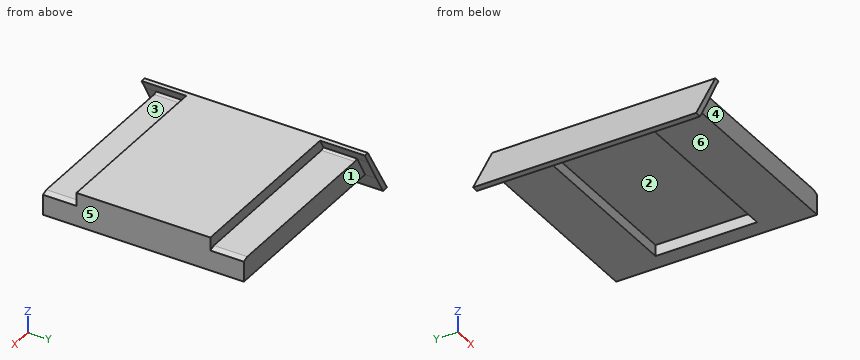
from build123d import *

# Parameters (mm, degrees)
F1_DEPTH  = 20
F3_DEPTH  = 4
F5_DEPTH  = 1
F7_DEPTH  = 20.001
F10_W     = 15
F10_H     = 9.1
F11_DEPTH = 1


# Not quite as in the source:
# - a pattern or mirror of a feature is missing from the dataset's text; its kind, count and spacing are read off the source's solid


with BuildPart() as f1:
    # F0 (on Front) → F1 (new body)
    with BuildSketch(Plane.XZ):
        Polygon((-16.45, 3), (-19.25, -1.7), (-18.09, -1.7), (-17.0772340426, 0), (0, 0), (0, 3), align=None)
    extrude(amount=F1_DEPTH)

    # F2 (on face) → F3 (cut)
    with BuildSketch(Plane.XZ.offset(20)):
        Polygon((-16.2, 2), (-0.5, 2), (0, 1.8180148829), (0, 3), (-16, 3), (-16.5, 2.1091910703), align=None)
    f3 = extrude(amount=-F3_DEPTH, mode=Mode.SUBTRACT)

    # F3_copies: F3 across plane
    add(f3.mirror(Plane.ZX.offset(-10)), mode=Mode.SUBTRACT)

    # F4 (on face) → F5 (cut)
    with BuildSketch(Plane.XZ.offset(20)):
        Polygon((0, 0), (0, 1.8180148829), (-0.5, 2), (-16.2, 2), (-16.5, 2.1091910703), (-17.683862779, 0), align=None)
    f5 = extrude(amount=-F5_DEPTH, mode=Mode.SUBTRACT)

    # F5_copies: F5 across plane
    add(f5.mirror(Plane.ZX.offset(-10)), mode=Mode.SUBTRACT)

    # F6 (on face) → F7 (cut, through all)
    with BuildSketch(Plane.XZ.offset(20)):
        Polygon((-18.67, -1.7), (-18.09, -1.7), (-17.0772340426, 0), (-17.683862779, 0), align=None)
    extrude(amount=-F7_DEPTH, mode=Mode.SUBTRACT)

    # F10 (on face) → F11 (cut)
    with BuildSketch(Plane(origin=(0, 0, 0), x_dir=(1, 0, 0), z_dir=(0, 0, -1))):
        with Locations((-9, 10)):
            Rectangle(F10_W, F10_H)
    extrude(amount=-F11_DEPTH, mode=Mode.SUBTRACT)


solid = f1.part
Could you check a few things on this model? Use its own coordinates, in mm. Face numbers are marked on the shaded views. A direction names the side the tool comes from. Coordinates: 2 decimals unless noted, no trailing zeros. Write each loop counter-clockwise with the first axis right and the second up, starting at its lowest first coordinate (ties: lowest second). Pieces come first, ordered by that corner, then holes. Notation, with made-up numbers: (-20, 65) - (-9, 65) arc R17 cw to (-9, 92) - close; hole circle Ø8 at (18.5, -39.5). An arc over 180 degrees is marked (long way). Write item = value, one per line.
1) For the marked faces 5 and 6, which set-ups out of +Z, -Z, +X, -X, +Y, -Y let a thin tool reach every point of the face, with its end or its side?
Result set:
face_5 = +Z, -Z, +X, +Y, -Y
face_6 = -Z, +X, +Y, -Y
2) Suppose I cut it at B-B on x = -8.75. Please give me the cut outline in (y, z).
Result set:
outline = (-19, 0) - (-14.55, 0) - (-14.55, 1) - (-5.45, 1) - (-5.45, 0) - (-1, 0) - (-1, 2) - (-4, 2) - (-4, 3) - (-16, 3) - (-16, 2) - (-19, 2) - close
3) Will these pins go through, and if not, where does the flat tip stop? pin 1 Ø2.5 at (x, y) = (-9, -8) entering from -Z; pin 2 Ø2.5 at (x, z) = (-10, 0.5) entering from +Y; pin 3 Ø0.6 at (x, z) = (-6.5, 2.5) entering from -Y.
Result set:
pin_1 = 1
pin_2 = -1
pin_3 = -16
4) We'd pull the mould along Y, two halves only. Please class the marked faces 1, 2, 3 and 4: +Y half, -Y half, draft (parallel to the pull), parting line (faces both ways), or undercut.
Result set:
face_1 = +Y half
face_2 = undercut
face_3 = draft
face_4 = -Y half
5) Suppose I cut it at A-A on y = -7.25. Please give me the cut outline in (x, z), plus the area to 3 significant figures.
Result set:
outline = (-19.25, -1.7) - (-18.67, -1.7) - (-17.68, 0) - (-16.5, 0) - (-16.5, 1) - (-1.5, 1) - (-1.5, 0) - (0, 0) - (0, 3) - (-16.45, 3) - close
area = 38.0 mm2
6) Suppose I cut it at D-D on z = -0.5. Please give me the cut outline in (x, y).
Result set:
outline = (-18.54, -20) - (-17.97, -20) - (-17.97, 0) - (-18.54, 0) - close
7) Please list where these lines run through material, in increasing order: line 1 (Z direction, x = -11.25, y = -17.75); line 2 (Y direction, x = -4.25, z = 1.9); line 3 (Y direction, x = -5.75, z = 2.55). Write a range as [from, to].
Result set:
line_1 = [0, 2]
line_2 = [-19, -1]
line_3 = [-16, -4]
8) Suppose I cut it at C-C on x = -1. Please give me the cut outline in (y, z).
Result set:
outline = (-19, 0) - (-1, 0) - (-1, 2) - (-4, 2) - (-4, 3) - (-16, 3) - (-16, 2) - (-19, 2) - close
